from build123d import *

# Parameters (mm, degrees)
SKETCH1_W               = 28.2
SKETCH1_H               = 28.2
BOSS_EXTRUDE1_DEPTH     = 33
SKETCH2_R               = 11.5
BOSS_EXTRUDE2_DEPTH     = 2
SKETCH3_R               = 2.5
BOSS_EXTRUDE3_DEPTH     = 19
SKETCH4_R               = 1.25
CUT_EXTRUDE1_DEPTH      = 8
MIRROR2_COPY_1_SKETCH_R = 1.25
MIRROR2_COPY_1_DEPTH    = 8
SKETCH5_W               = 3
SKETCH5_H               = 3
CUT_EXTRUDE2_DEPTH      = 4
MIRROR4_COPY_1_SKETCH_W = 3
MIRROR4_COPY_1_SKETCH_H = 3
MIRROR4_COPY_1_DEPTH    = 4
SKETCH6_R               = 2.5
CUT_EXTRUDE3_DEPTH      = 4
FILLET1_R               = 2
FILLET2_R               = 1
FILLET3_R               = 1


with BuildPart() as part:
    # Sketch1 → Boss-Extrude1 (new body)
    with BuildSketch(Plane(origin=(0, 0, 0), x_dir=(1, 0, 0), z_dir=(0, 1, 0))):
        Rectangle(SKETCH1_W, SKETCH1_H)
    extrude(amount=BOSS_EXTRUDE1_DEPTH)

    # Sketch2 → Boss-Extrude2 (add)
    with BuildSketch(Plane(origin=(0, 33, 0), x_dir=(1, 0, 0), z_dir=(0, 1, 0))):
        Circle(SKETCH2_R)
    extrude(amount=BOSS_EXTRUDE2_DEPTH)

    # Sketch3 → Boss-Extrude3 (add)
    with BuildSketch(Plane(origin=(0, 35, 0), x_dir=(1, 0, 0), z_dir=(0, 1, 0))):
        Circle(SKETCH3_R)
    extrude(amount=BOSS_EXTRUDE3_DEPTH)

    # Sketch4 → Cut-Extrude1 (cut)
    with BuildSketch(Plane(origin=(0, 33, 0), x_dir=(1, 0, 0), z_dir=(0, 1, 0))):
        with Locations((-11.5, 11.5)):
            Circle(SKETCH4_R)
    cut_extrude1 = extrude(amount=-CUT_EXTRUDE1_DEPTH, mode=Mode.SUBTRACT)

    # Mirror1: Cut-Extrude1 across plane
    add(cut_extrude1.mirror(Plane(origin=(0, 0, 0), x_dir=(0, 0, 1), z_dir=(1, 0, 0))), mode=Mode.SUBTRACT)

    # Mirror2: Cut-Extrude1 across plane
    add(cut_extrude1.mirror(Plane.XY), mode=Mode.SUBTRACT)

    # Mirror2 copy 1 sketch → Mirror2 copy 1 (cut)
    with BuildSketch(Plane(origin=(0, 33, 0), x_dir=(-1, 0, 0), z_dir=(0, 1, 0))):
        with Locations((-11.5, 11.5)):
            Circle(MIRROR2_COPY_1_SKETCH_R)
    extrude(amount=-MIRROR2_COPY_1_DEPTH, mode=Mode.SUBTRACT)

    # Sketch5 → Cut-Extrude2 (cut)
    with BuildSketch(Plane.XZ):
        with Locations((-12.6, 12.6)):
            Rectangle(SKETCH5_W, SKETCH5_H)
    cut_extrude2 = extrude(amount=-CUT_EXTRUDE2_DEPTH, mode=Mode.SUBTRACT)

    # Mirror3: Cut-Extrude2 across plane
    add(cut_extrude2.mirror(Plane(origin=(0, 0, 0), x_dir=(0, 0, 1), z_dir=(1, 0, 0))), mode=Mode.SUBTRACT)

    # Mirror4: Cut-Extrude2 across plane
    add(cut_extrude2.mirror(Plane.XY), mode=Mode.SUBTRACT)

    # Mirror4 copy 1 sketch → Mirror4 copy 1 (cut)
    with BuildSketch(Plane(origin=(0, 0, 0), x_dir=(-1, 0, 0), z_dir=(0, -1, 0))):
        with Locations((-12.6, 12.6)):
            Rectangle(MIRROR4_COPY_1_SKETCH_W, MIRROR4_COPY_1_SKETCH_H)
    extrude(amount=-MIRROR4_COPY_1_DEPTH, mode=Mode.SUBTRACT)

    # Sketch6 → Cut-Extrude3 (cut)
    with BuildSketch(Plane.XZ):
        Circle(SKETCH6_R)
    extrude(amount=-CUT_EXTRUDE3_DEPTH, mode=Mode.SUBTRACT)

    # Fillet1
    fillet1_edges = [part.edges().sort_by_distance(p)[0] for p in [
        (14.1, 18.5, 14.1),
        (-14.1, 18.5, 14.1),
        (-14.1, 18.5, -14.1),
        (14.1, 18.5, -14.1),
    ]]
    fillet(fillet1_edges, radius=FILLET1_R)

    # Fillet2
    fillet2_edges = [part.edges().sort_by_distance(p)[0] for p in [
        (-14.1, 2, 11.1),
        (-11.1, 2, 14.1),
        (-11.1, 2, 11.1),
        (14.1, 2, 11.1),
        (11.1, 2, 11.1),
        (11.1, 2, 14.1),
        (-14.1, 2, -11.1),
        (-11.1, 2, -11.1),
        (-11.1, 2, -14.1),
        (14.1, 2, -11.1),
        (11.1, 2, -14.1),
        (11.1, 2, -11.1),
    ]]
    fillet(fillet2_edges, radius=FILLET2_R)

    # Fillet3
    fillet3_edges = [part.edges().sort_by_distance(p)[0] for p in [
        (-2.5, 54, 0),
    ]]
    fillet(fillet3_edges, radius=FILLET3_R)


solid = part.part
Could you check a few things on this model? Use its own coordinates, in mm. A direction names the side the tool comes from. Round coordinates to 2 decimals unless told otherwise and drop trailing zeros. Write each loop counter-clockwise with the first axis right and the second up, starting at its lowest first coordinate (ties: lowest second). Pieces come first, ordered by that corner, then holes. Notation, with made-up numbers: (1.25, 31.25) - (5.25, 31.25) arc R35 ccw to (5.25, 68.25) - close; hole circle Ø9 at (-4, 6). An arc over 180 degrees is marked (long way). Put each result on its own line as item: value. Start each with the question number.
(1) For faces 4 (the flat face through (-13, 4, 13)), 5 (the flat face through (13, 4, -13)), 6 (the flat face through (13, 4, 13)), 7 (the cylindrical face through (-12.421, 29.056, -12.345)), which set-ups out of +Z, -Z, +X, -X, +Y, -Y let a thin tool reach every point of the face, with its end or its side?
(2) I want a section at C-C, the plane x = 9. Please give me the cut outline in (y, z).
(3) I want a section at B-B, the plane z = 0. Please give me the cut outline in (x, y), plus the area to 3 significant figures.
(4) I need wall thicknesses on probe 1 along Z at (x, y) = (-11.5, 27); probe 2 along Z at (x, y) = (0, 2.75); probe 3 along Y at (x, z) = (-1, 4.5). Which ranges of each line are inside material? Lowest first, please.
(5) Will these pins go through, and if not, where does the flat tip stop? pin 1 (3 mm diameter, centred on x = -11.5, z = -11.5, fed in from +Y); pin 2 (0.8 mm diameter, centred on x = 12.5, y = 1.5, fed in from -Z); pin 3 (2 mm diameter, centred on x = 11.5, z = 11.5, fed in from +Y).
(6) I want a section at D-D, the plane y = 43. Please give me the cut outline in (x, z).
(7) Thinking about a two-plate mould opening in X: for faces 1 (the cylindrical face through (12.421, 29.056, -12.345)), 2 (the flat face through (0, 16, 14.1)), 3 (the cylindrical face through (-0.54, 43.87, 2.44)), which applies, released by +X, released by -X, zero draft, split by the parting line, or undercut?
(8) I want a section at A-A, the plane y = 30.5. Please give me the cut outline in (x, z), plus the area to 3 significant figures.
Here are the results:
1. face 4: +Z, -X, -Y
1. face 5: -Z, +X, -Y
1. face 6: +Z, +X, -Y
1. face 7: +Y
2. outline: (0, -14.1) - (33, -14.1) - (33, -7.16) - (35, -7.16) - (35, 7.16) - (33, 7.16) - (33, 14.1) - (0, 14.1) - close
3. outline: (-14.1, 0) - (-2.5, 0) - (-2.5, 4) - (2.5, 4) - (2.5, 0) - (14.1, 0) - (14.1, 33) - (11.5, 33) - (11.5, 35) - (2.5, 35) - (2.5, 53) arc R1 ccw to (1.5, 54) - (-1.5, 54) arc R1 ccw to (-2.5, 53) - (-2.5, 35) - (-11.5, 35) - (-11.5, 33) - (-14.1, 33) - close
3. area: 1,050 mm^2
4. probe 1: z = -14.1 to -12.75, -10.25 to 10.25, 12.75 to 14.1
4. probe 2: z = -14.1 to -2.5, 2.5 to 14.1
4. probe 3: y = 0 to 35
5. pin 1: stops at y = 33
5. pin 2: stops at z = -11.1
5. pin 3: stops at y = 25
6. outline: circle Ø5 at (0, 0)
7. face 1: undercut
7. face 2: zero draft
7. face 3: split by the parting line
8. outline: (-14.1, -12.1) arc R2 ccw to (-12.1, -14.1) - (12.1, -14.1) arc R2 ccw to (14.1, -12.1) - (14.1, 12.1) arc R2 ccw to (12.1, 14.1) - (-12.1, 14.1) arc R2 ccw to (-14.1, 12.1) - close; hole circle Ø2.5 at (-11.5, -11.5); hole circle Ø2.5 at (-11.5, 11.5); hole circle Ø2.5 at (11.5, -11.5); hole circle Ø2.5 at (11.5, 11.5)
8. area: 772 mm^2
